Drawing for the job (mm, zero at the part's lowest x, y, z). A direction names the side the tool comes from. Coordinates: 2 decimals unless noted, no trailing zeros. Order: outer loops, then holes, each group sorted by start corner. A loop starts at its lowest first (then second) coordinate and runs counter-clockwise, first axis right, second up.
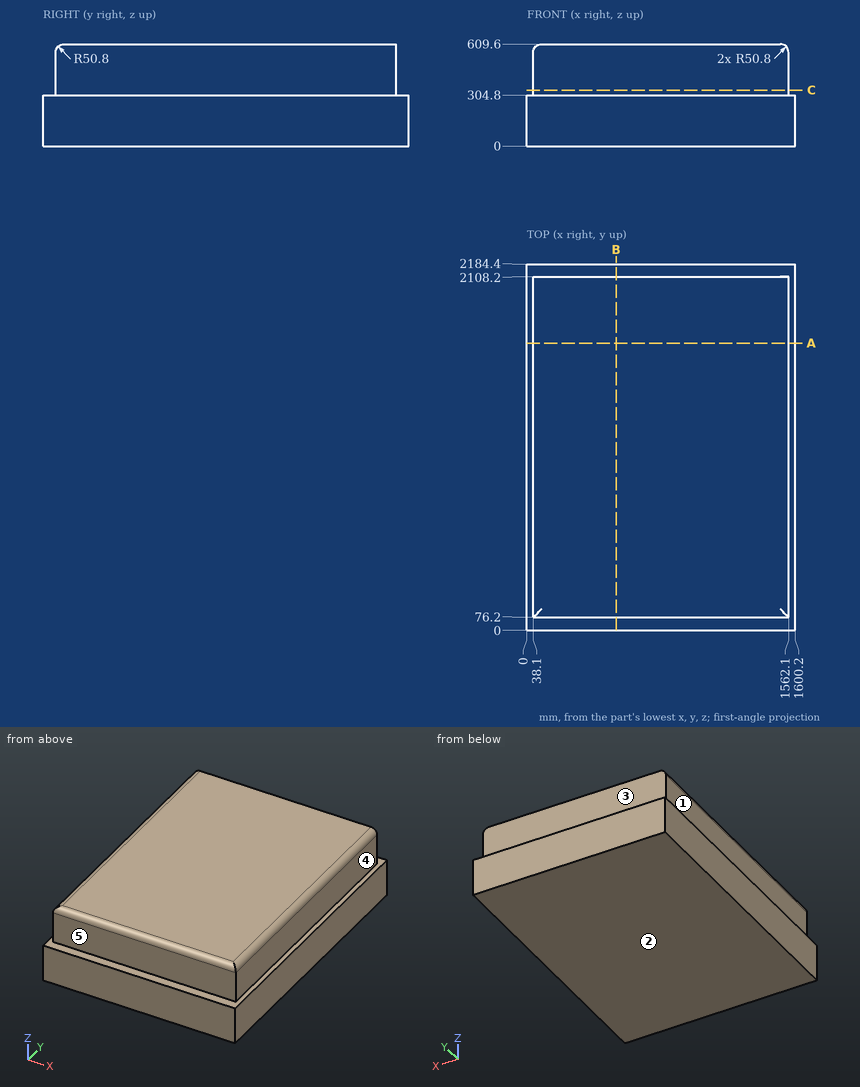
(1) Slice it at B-B, the plane x = 532. Give the cut face in (y, z), then the cut area to 3 significant figures.
(2) Probe line 1 (Y direction, x = 1022, z = 316); line 2 (X direction, y = 1587, z = 323); line 3 (X direction, y = 452, z = 573.5). List the from-to ranges inside material, lowest first.
(3) Slice it at C-C, the plane z = 335. Give the cut face in (x, y).
(4) Tool access for the marked faces 1, 2, 3, 4 and 5: list every direction of +Z, -Z, +X, -X, +Y, -Y with a clear straight run to the whole face (end or side of a thin tool).
(5) Drop flat-ended pins along their axis: pin 1 (1 mm diameter, centred on y = 1562, z = 487, fed in from +X); pin 2 (3 mm diameter, centred on x = 270.5, z = 522.5, fed in from +Y). Give the stop position or say it passes through.
(6) Slice it at A-A, the plane y = 1713. Give the cut face in (x, z), then the cut area to 3 significant figures.
Here are the results:
1. outline: (0, 0) - (2184.4, 0) - (2184.4, 304.8) - (2108.2, 304.8) - (2108.2, 609.6) - (127, 609.6) arc R50.8 ccw to (76.2, 558.8) - (76.2, 304.8) - (0, 304.8) - close
1. area: 1,280,000 mm2
2. line 1: y = 76.2 to 2108.2
2. line 2: x = 38.1 to 1562.1
2. line 3: x = 40.27 to 1559.93
3. outline: (38.1, 76.2) - (1562.1, 76.2) - (1562.1, 2108.2) - (38.1, 2108.2) - close
4. face 1: +Z, -X, +Y, -Y
4. face 2: -Z, +X, -X, +Y, -Y
4. face 3: +Z, +X, -X, +Y
4. face 4: +Z, +X, +Y, -Y
4. face 5: +Z, +X, -X, -Y
5. pin 1: stops at x = 1562.1
5. pin 2: stops at y = 2108.2
6. outline: (0, 0) - (1600.2, 0) - (1600.2, 304.8) - (1562.1, 304.8) - (1562.1, 558.8) arc R50.8 ccw to (1511.3, 609.6) - (88.9, 609.6) arc R50.8 ccw to (38.1, 558.8) - (38.1, 304.8) - (0, 304.8) - close
6. area: 951,000 mm2
